Could you check a few things on this model? Use its own coordinates, in mm. A direction names the side the tool comes from. Give positions to 0.01 mm unless a question says otherwise; leave off trailing zeros. Loops run counter-clockwise (first coordinate to the right, second up) from the corner with the lowest first, then second, coordinate; pieces in that order, holes last. Notation, with made-up numbers: (85.25, 3.5) - (94.25, 3.5) arc R20 cw to (94.25, 30.5) - close; hole circle Ø6 at (-1.5, 46.5). An arc over 180 degrees is marked (long way). One line per item, written item: value. Start each with the question number.
Q1. I'm going to push flat-ended pins straight in: P1, Ø5, axis at x = -3.5, z = 300, coming from the +Y side; P2, Ø8, axis at y = 690, z = 18.5, coming from the -X side; P3, Ø16, axis at x = 18.5, y = 510, coming from the -Z side; P4, Ø13, axis at y = 270, z = 18.5, coming from the +X side. Where does each tip first touch, or does it pass through?
Q2. I want a section at A-A (x = 234). Please give me the cut outline in (y, z).
Q3. I want a section at B-B (z = 239.5). Please give me the cut outline in (x, y), then the cut area to 3 significant figures.
Q4. For faces 1 (the face through (2, 40, -11)), 2 (the face through (25, 40, 25)), 3 (the face through (-5, 65, 75)), which set-ups out of +Z, -Z, +X, -X, +Y, -Y let a thin tool reach every point of the face, with its end or its side?
Q5. If I drill on line 1 (X direction, y = 180, z = -5.5); line 2 (X direction, y = 3.5, z = 380), over which ranges is the centre line in solid material (lowest first)? Write a range as from..to.
```python
from build123d import *

# Parameters (mm, degrees)
EXTRUDE_2_DEPTH          = 10
EXTRUDE_3_DEPTH          = 40
EXTRUDE_4_DEPTH          = 700
SKETCH_13_W              = 60
SKETCH_13_H              = 60
EXTRUDE_7_DEPTH          = 30
EXTRUDE_1_DEPTH          = 40
EXTRUDE_8_DEPTH          = 10
EXTRUDE_9_DEPTH          = 10
SKETCH_36_R              = 5
CUT_EXTRUDE_1_DEPTH      = 10
PATTERN_LINEAR_1_COUNT   = 20
PATTERN_LINEAR_1_PITCH   = 30
SKETCH_37_R              = 5
CUT_EXTRUDE_2_DEPTH      = 10
PATTERN_LINEAR_2_COUNT   = 20
PATTERN_LINEAR_2_PITCH   = 30
CUT_EXTRUDE_3_DEPTH      = 901
CUT_EXTRUDE_3_DEPTH_BACK = 901
SKETCH_38_R              = 5
SKETCH_39_W              = 10
SKETCH_39_H              = 15
CUT_EXTRUDE_4_DEPTH      = 40
SKETCH_40_W              = 10
SKETCH_40_H              = 15
CUT_EXTRUDE_5_DEPTH      = 40


# Read off the part's stored shape, not the designer's step: 拉伸-薄壁1
with BuildPart() as part:
    # 草图3 → 凸台-拉伸2 (new body)
    with BuildSketch(Plane(origin=(0, 0, 0), x_dir=(1, 0, 0), z_dir=(0, 1, 0))):
        Polygon((0, 0), (0, -400), (50, -400), (50, -50), (400, -50), (400, 0), align=None)
    extrude(amount=EXTRUDE_2_DEPTH)

    # 草图4 → 凸台-拉伸3 (add)
    with BuildSketch(Plane(origin=(0, 0, 0), x_dir=(1, 0, 0), z_dir=(0, 1, 0))):
        Polygon((0, -400), (-10, -400), (-10, 10), (400, 10), (400, 0), (0, 0), align=None)
    extrude(amount=EXTRUDE_3_DEPTH)

    # 草图6 → 凸台-拉伸4 (add)
    with BuildSketch(Plane(origin=(0, 10, 0), x_dir=(1, 0, 0), z_dir=(0, 1, 0))):
        Polygon((-10, 10), (-10, -50), (0, -50), (0, 0), (50, 0), (50, 10), align=None)
    extrude(amount=EXTRUDE_4_DEPTH)

    # 草图13 → 凸台-拉伸7 (add)
    with BuildSketch(Plane(origin=(0, 10, 0), x_dir=(1, 0, 0), z_dir=(0, 1, 0))):
        with Locations((20, -20)):
            Rectangle(SKETCH_13_W, SKETCH_13_H)
    extrude(amount=EXTRUDE_7_DEPTH)

    # 拉伸-薄壁1 outline → 拉伸-薄壁1 (add)
    with BuildSketch(Plane(origin=(0, 0, 0), x_dir=(1, 0, 0), z_dir=(0, 1, 0))):
        with BuildLine():
            Line((-10, 10), (50, 10))
            Line((50, 10), (50, 20))
            Line((50, 20), (-10, 20))
            ThreePointArc((-10, 20), (-17.071067812, 17.071067812), (-20, 10))
            Line((-20, 10), (-20, -50))
            Line((-20, -50), (-10, -50))
            Line((-10, -50), (-10, 10))
        make_face()
    extrude(amount=EXTRUDE_1_DEPTH)

    # 草图34 → 凸台-拉伸8 (add)
    with BuildSketch(Plane(origin=(0, 0, -10), x_dir=(-1, 0, 0), z_dir=(0, 0, -1))):
        Polygon((-100, 40), (-50, 90), (-50, 40), align=None)
    extrude(amount=-EXTRUDE_8_DEPTH)

    # 草图35 → 凸台-拉伸9 (add)
    with BuildSketch(Plane.ZY.offset(10)):
        Polygon((50, 90), (50, 40), (100, 40), align=None)
    extrude(amount=-EXTRUDE_9_DEPTH)

    # 草图36 → 切除-拉伸1 (cut)
    with BuildSketch(Plane(origin=(0, 0, 0), x_dir=(0, 0, -1), z_dir=(1, 0, 0))):
        with Locations((-18.5, 690)):
            Circle(SKETCH_36_R)
    cut_extrude_1 = extrude(amount=-CUT_EXTRUDE_1_DEPTH, mode=Mode.SUBTRACT)

    # 阵列(线性)1: 切除-拉伸1 ×20
    with Locations(*[(0, -i * PATTERN_LINEAR_1_PITCH, 0) for i in range(1, PATTERN_LINEAR_1_COUNT)]):
        add(cut_extrude_1, mode=Mode.SUBTRACT)

    # 草图37 → 切除-拉伸2 (cut)
    with BuildSketch(Plane.XY):
        with Locations((18.5, 690)):
            Circle(SKETCH_37_R)
    cut_extrude_2 = extrude(amount=-CUT_EXTRUDE_2_DEPTH, mode=Mode.SUBTRACT)

    # 阵列(线性)2: 切除-拉伸2 ×20
    with Locations(*[(0, -i * PATTERN_LINEAR_2_PITCH, 0) for i in range(1, PATTERN_LINEAR_2_COUNT)]):
        add(cut_extrude_2, mode=Mode.SUBTRACT)

    # 草图38 → 切除-拉伸3 (cut, two sides: drawn at the far end of the back side and taken through both)
    with BuildSketch(Plane(origin=(0, 10, 0), x_dir=(1, 0, 0), z_dir=(0, 1, 0)).offset(-CUT_EXTRUDE_3_DEPTH_BACK)):
        with Locations(Location((25, -380, 0), (0, 0, 270))):
            Circle(SKETCH_38_R)
        with Locations(Location((380, -25, 0), (0, 0, 270))):
            Circle(SKETCH_38_R)
    extrude(amount=CUT_EXTRUDE_3_DEPTH + CUT_EXTRUDE_3_DEPTH_BACK, mode=Mode.SUBTRACT)

    # 草图39 → 切除-拉伸4 (cut)
    with BuildSketch(Plane.XY.offset(400)):
        with Locations((-5, 17.5)):
            Rectangle(SKETCH_39_W, SKETCH_39_H)
    extrude(amount=-CUT_EXTRUDE_4_DEPTH, mode=Mode.SUBTRACT)

    # 草图40 → 切除-拉伸5 (cut)
    with BuildSketch(Plane(origin=(400, 0, 0), x_dir=(0, 0, -1), z_dir=(1, 0, 0))):
        with Locations((5, 17.5)):
            Rectangle(SKETCH_40_W, SKETCH_40_H)
    extrude(amount=-CUT_EXTRUDE_5_DEPTH, mode=Mode.SUBTRACT)


solid = part.part
```
Worked answers:
1. P1: stops at y = 40
1. P2: passes through
1. P3: stops at z = -10
1. P4: stops at x = 0
2. outline: (0, -10) - (40, -10) - (40, 0) - (10, 0) - (10, 50) - (0, 50) - close
3. outline: (-10, 0) - (50, 0) - (50, 10) - (0, 10) - (0, 40) - (-10, 40) - close
3. area: 900 mm²
4. face 1: -Z, -X, +Y
4. face 2: +Z, +X, +Y
4. face 3: +Z, +X, -X, +Y
5. line 1: x = -10..13.5, 23.5..50
5. line 2: x = -10..20, 30..50
